Job drawing, mm, ordinate dimensions from the low corner. One solid piece. A direction names the side the tool comes from. Give positions to 0.01 mm unless a question says otherwise; leave off trailing zeros. Order: outer loops, then holes, each group sorted by start corner. A loop starts at its lowest first (then second) coordinate and runs counter-clockwise, first axis right, second up.
Item 1: Which spindle directions (+Z, -Z, +X, -X, +Y, -Y) get a long thin tool onto all of the face, cutting with end or side? Do the marked faces 4 and 5. Say none if no direction does.
Item 2: Band-saw the part on C-C on x = 8. Give the cut face in (y, z), plus the area to 3 significant figures.
Item 3: Band-saw the part on A-A on z = 3. Give the cut face in (x, y).
Item 4: Wall check: L1, parallel to Z at x = 8, y = 6.25; L2, parallel to Z at x = 10, y = 4.5; L3, parallel to Y at x = 8, z = 3. Give the ranges that are in metal, low to high.
Item 5: Flat gauge pins, fed straight in: P1, Ø4, axis at y = 3, z = 3, coming from the -X side; P2, Ø1.5, axis at x = 1, y = 4.5, coming from the -Z side. Where does each tip first touch, or does it go through?
Item 6: Band-saw the part on B-B on y = 5. Give the cut face in (x, z).
Item 7: Band-saw the part on D-D on x = 4.5. Give the cut face in (y, z), plus the area to 3 significant figures.
Item 8: Two-plate mould, pull along Y, no slides. Class the marked faces 1, 2 and 3: released by +Y, released by -Y, zero draft, split by the parting line, or undercut.
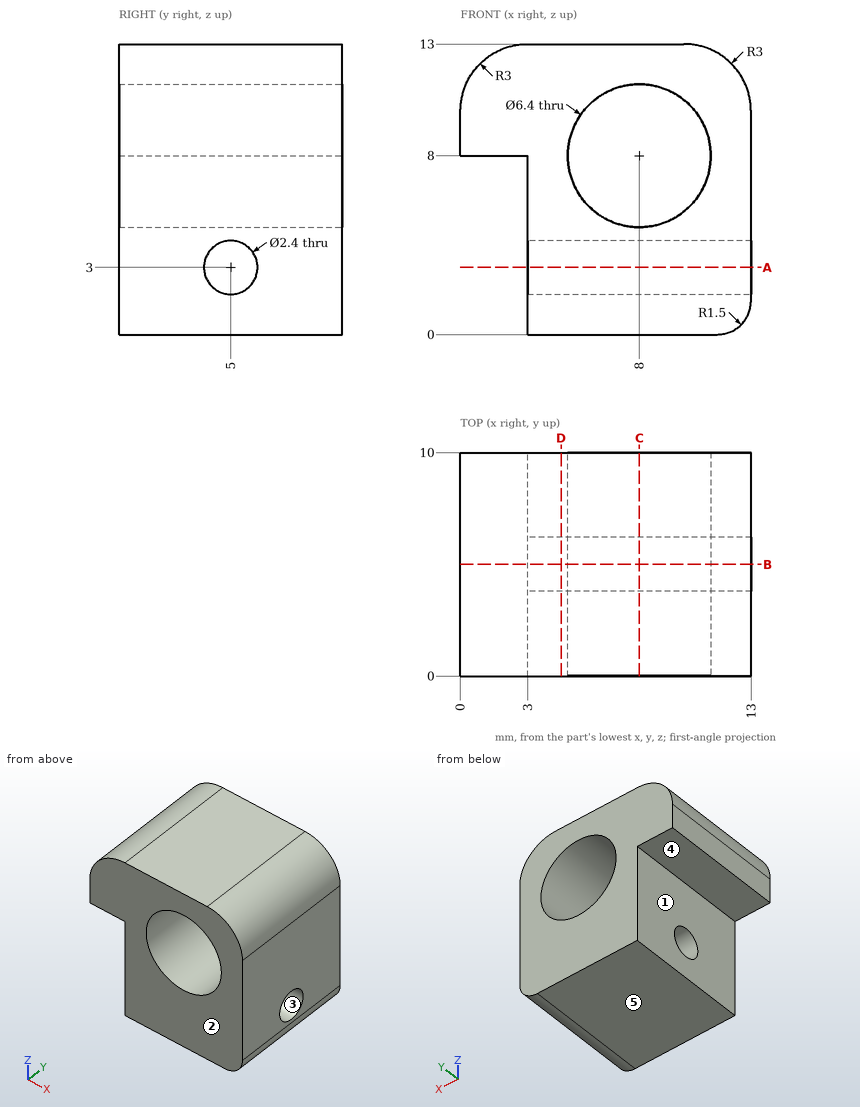
The answers:
1. face 4: -Z, -X, +Y, -Y
1. face 5: -Z, +X, -X, +Y, -Y
2. outline: (0, 0) - (10, 0) - (10, 4.8) - (0, 4.8) - close; (0, 11.2) - (10, 11.2) - (10, 13) - (0, 13) - close; hole circle Ø2.4 at (5, 3)
2. area: 61.5 mm2
3. outline: (3, 0) - (13, 0) - (13, 3.8) - (3, 3.8) - close; (3, 6.2) - (13, 6.2) - (13, 10) - (3, 10) - close
4. L1: z = 0 to 4.8, 11.2 to 13
4. L2: z = 0 to 1.91, 4.09 to 5.5, 10.5 to 13
4. L3: y = 0 to 3.8, 6.2 to 10
5. P1: stops at x = 3
5. P2: stops at z = 8
6. outline: (0, 8) - (3, 8) - (3, 4.2) - (13, 4.2) - (13, 10) arc R3 ccw to (10, 13) - (3, 13) arc R3 ccw to (0, 10) - close; (3, 0) - (11.5, 0) arc R1.5 ccw to (13, 1.5) - (13, 1.8) - (3, 1.8) - close; hole circle Ø6.4 at (8, 8)
7. outline: (0, 0) - (10, 0) - (10, 13) - (0, 13) - close; hole circle Ø2.4 at (5, 3)
7. area: 125 mm2
8. face 1: zero draft
8. face 2: released by -Y
8. face 3: undercut
